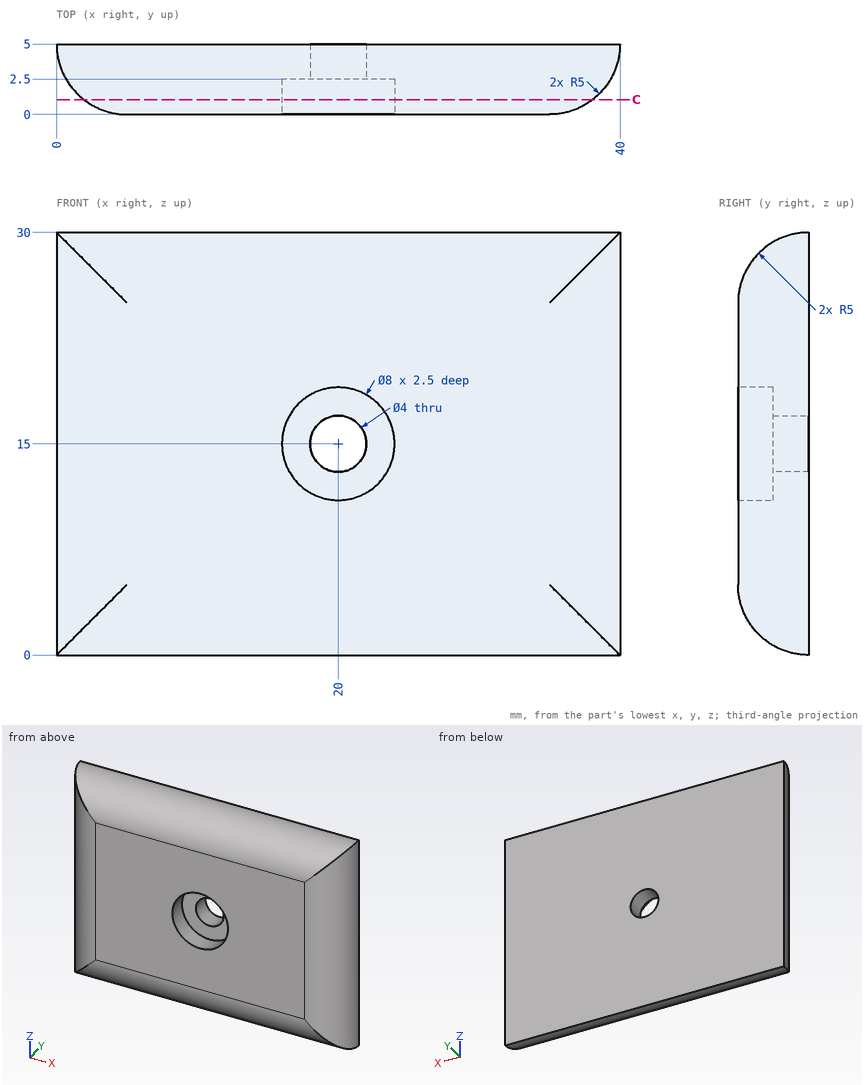
Print and shaded views of the part. All mm, measured from the part's lowest x, y and z. Coordinates: 2 decimals unless noted, no trailing zeros. Order: outer loops, then holes, each group sorted by start corner. A loop starts at its lowest first (then second) coordinate and runs counter-clockwise, first axis right, second up. Notation, with made-up numbers: (81, 35) - (87, 35) arc R8 cw to (87, 49) - close; hole circle Ø8 at (25.25, -33). An arc over 180 degrees is marked (long way). Return JSON: item names as keys, results as strings. Group by question number.
Item 1: Drill centre lines: probe 1 along Y at (x, z) = (16.5, 16.5); probe 2 along X at (y, z) = (4.35, 15); probe 3 along X at (y, z) = (0.5, 17.5). Where is each one in solid material? Low to high. Write a range as from..to.
Item 2: Pin check, flat tips, straight feed: pin 1 (1.5 mm diameter, centred on y = 3, z = 12, fed in from -X); pin 2 (4.5 mm diameter, centred on x = 20, z = 15, fed in from -Y); pin 3 (2 mm diameter, centred on x = 15.5, y = 1, fed in from -Z). Stop position of each tip, or through.
Item 3: Cut at C-C (y = 1.05). List the corners of the cut face in (x, z).
Check values:
{
 "1": {"probe 1": "y = 2.5..5", "probe 2": "x = 0.04..18, 22..39.96", "probe 3": "x = 2.82..16.88, 23.12..37.18"},
 "2": {"pin 1": "stops at x = 0.16", "pin 2": "stops at y = 2.5", "pin 3": "stops at z = 1"},
 "3": {"outline": "(1.93, 1.93) - (38.07, 1.93) - (38.07, 28.07) - (1.93, 28.07) - close; hole circle Ø8 at (20, 15)"}
}
